Verification items for this drawing (mm, ordinates from the low corner). A direction names the side the tool comes from. Round coordinates to 2 decimals unless told otherwise and drop trailing zeros. Loops run counter-clockwise (first coordinate to the right, second up) from the corner with the lowest first, then second, coordinate; pieces in that order, holes last. Notation, with made-up numbers: (77, 87.5) - (119, 87.5) arc R27 ccw to (119, 103.5) - close; hole circle Ø4 at (54, -32). An arc over 180 degrees is marked (long way). Put each result on its own line as item: value.
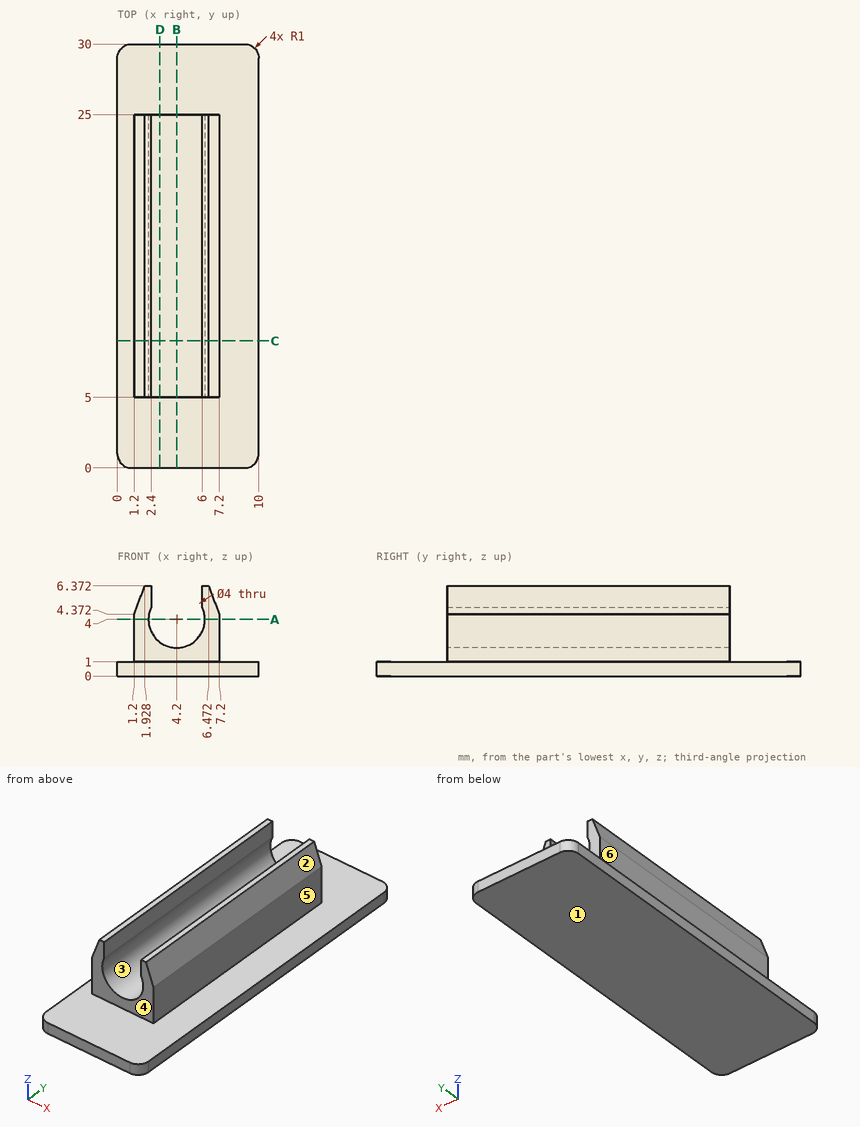
Item 1: Go/stop test with flat-tipped pins: pin 1 (2.5 mm diameter, centred on x = 5, z = 2.5, fed in from -Y); pin 2 (1.2 mm diameter, centred on y = 16.5, z = 5.5, fed in from +X); pin 3 (1.2 mm diameter, centred on y = 17, z = 6, fed in from -X); pin 4 (3.5 mm diameter, centred on y = 17.5, z = 2.5, fed in from -X). Record where each tip stops, or that it passes through.
Filled sheet:
pin 1: y = 5
pin 2: x = 7.01
pin 3: x = 1.57
pin 4: x = 0
Item 2: Section check A-A on z = 4. Enter the section's corners in (x, y).
Filled sheet:
outline: (1.2, 5) - (2.2, 5) - (2.2, 25) - (1.2, 25) - close; (6.2, 5) - (7.2, 5) - (7.2, 25) - (6.2, 25) - close
Item 3: Section check B-B on x = 4.2. Enter the section's corners in (y, z).
Filled sheet:
outline: (0, 0) - (30, 0) - (30, 1) - (25, 1) - (25, 2) - (5, 2) - (5, 1) - (0, 1) - close
Item 4: Tool access check on the marked faces 5 and 6. Record the directions out of +Z, -Z, +X, -X, +Y, -Y that give a thin tool (end or side, any length) a straight path to the whole face; none if there is none.
Filled sheet:
face 5: +Z, +X, +Y, -Y
face 6: +Z, -X, +Y, -Y
Item 5: Thickness scan on line 1 (X direction, y = 19, z = 4); line 2 (Y direction, x = 2, z = 4.75); line 3 (Z direction, x = 4.2, y = 15.25). Record the ranges inside material, lowest first. Write a range as from..to.
Filled sheet:
line 1: 1.2..2.2, 6.2..7.2
line 2: 5..25
line 3: 0..2
Item 6: Release check for a two-part mould opening along Z. For the marked faces 1, 2, 3 and 4 record: +Z half, -Z half, draft (parallel to the pull), parting line (faces both ways), or undercut.
Filled sheet:
face 1: -Z half
face 2: +Z half
face 3: undercut
face 4: draft
Item 7: Section check D-D on x = 3. Enter the section's corners in (y, z), then the cut area to 3 significant figures.
Filled sheet:
outline: (0, 0) - (30, 0) - (30, 1) - (25, 1) - (25, 2.4) - (5, 2.4) - (5, 1) - (0, 1) - close
area: 58.0 mm²
Item 8: Section check C-C on y = 9. Enter the section's corners in (x, z).
Filled sheet:
outline: (0, 0) - (10, 0) - (10, 1) - (7.2, 1) - (7.2, 4.37) - (6.47, 6.37) - (6, 6.37) - (6, 4.87) arc R2 cw (long way) to (2.4, 4.87) - (2.4, 6.37) - (1.93, 6.37) - (1.2, 4.37) - (1.2, 1) - (0, 1) - close
